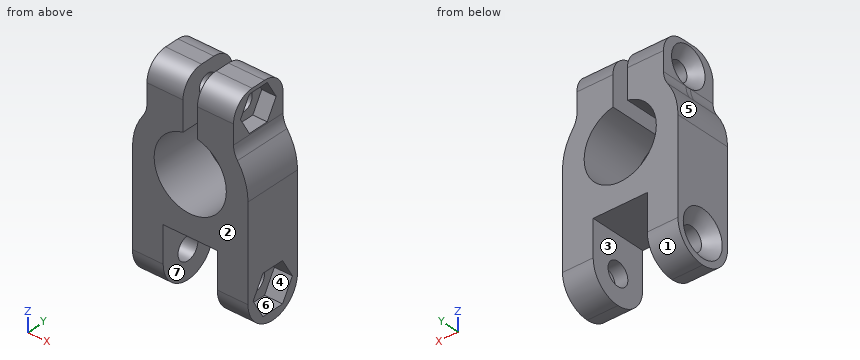
```python
from build123d import *

# Parameters (mm, degrees)
F1_DEPTH = 4
F2_R     = 1.35
F3_DEPTH = 14.001
F4_DEPTH = 2
F5_R     = 1.6
F6_DEPTH = 25
F7_DEPTH = 2.5
F8_SIZE  = 1.35
F9_R     = 3
F10_R    = 3.99999
F11_SIZE = 1.55


# Not quite as in the source:
# - a fillet or chamfer is up to 0.001 mm smaller than in the source, because OpenCascade refuses the exact size
# - a feature names something its author has since deleted; it is built from what else it names


with BuildPart() as f1:
    # F0 (on Front) → F1 (new body, symmetric)
    with BuildSketch(Plane.XZ):
        with BuildLine():
            ThreePointArc((1, 4.8989794856), (0, -5), (-1, 4.8989794856))
            Line((-1, 4.8989794856), (-1, 12))
            Line((-1, 12), (-6, 12))
            Line((-6, 12), (-6, 5.2915026221))
            ThreePointArc((-6, 5.2915026221), (-7.4833147735, 2.8284271247), (-8, 0))
            Line((-8, 0), (-8, -17))
            Line((-8, -17), (-3.75, -17))
            Line((-3.75, -17), (-3.75, -8))
            Line((-3.75, -8), (3.75, -8))
            Line((3.75, -8), (3.75, -17))
            Line((3.75, -17), (8, -17))
            Line((8, -17), (8, 0))
            ThreePointArc((8, 0), (7.4833147735, 2.8284271247), (6, 5.2915026221))
            Line((6, 5.2915026221), (6, 12))
            Line((6, 12), (1, 12))
            Line((1, 12), (1, 4.8989794856))
        make_face()
    extrude(amount=F1_DEPTH, both=True)

    # F2 (on face) → F3 (cut, through all)
    with BuildSketch(Plane.YZ.offset(6)):
        with Locations((0, 9)):
            Circle(F2_R)
    extrude(amount=-F3_DEPTH, mode=Mode.SUBTRACT)

    # F2 (on face) → F4 (cut)
    with BuildSketch(Plane.YZ.offset(6)):
        Polygon((2.8867513459, 9), (1.443375673, 11.5), (-1.443375673, 11.5), (-2.8867513459, 9), (-1.443375673, 6.5), (1.443375673, 6.5), align=None)
        with Locations((0, 9)):
            Circle(F2_R, mode=Mode.SUBTRACT)
    extrude(amount=-F4_DEPTH, mode=Mode.SUBTRACT)

    # F5 (on face) → F6 (cut)
    with BuildSketch(Plane.YZ.offset(8)):
        with Locations((0, -13)):
            Circle(F5_R)
    extrude(amount=-F6_DEPTH, mode=Mode.SUBTRACT)

    # F5 (on face) → F7 (cut)
    with BuildSketch(Plane.YZ.offset(8)):
        Polygon((1.5877132403, -10.25), (-1.5877132403, -10.25), (-3.1754264805, -13), (-1.5877132403, -15.75), (1.5877132403, -15.75), (3.1754264805, -13), align=None)
        with Locations((0, -13)):
            Circle(F5_R, mode=Mode.SUBTRACT)
    extrude(amount=-F7_DEPTH, mode=Mode.SUBTRACT)

    # F8
    f8_edges = [f1.edges().sort_by_distance(p)[0] for p in [
        (-6, -1.35, 9),
    ]]
    chamfer(f8_edges, length=F8_SIZE)

    # F9
    f9_edges = [f1.edges().sort_by_distance(p)[0] for p in [
        (-3.5, -4, 12),
        (3.5, -4, 12),
        (3.5, 4, 12),
        (-3.5, 4, 12),
        (6, 0, 5.291503),
        (-6, 0, 5.291503),
    ]]
    fillet(f9_edges, radius=F9_R)

    # F10 (radius 4 in the source; OpenCascade refuses exactly that, so slightly less here)
    f10_edges = [f1.edges().sort_by_distance(p)[0] for p in [
        (5.875, -4, -17),
        (-5.875, -4, -17),
        (-5.875, 4, -17),
        (5.875, 4, -17),
    ]]
    fillet(f10_edges, radius=F10_R)

    # F11
    f11_edges = [f1.edges().sort_by_distance(p)[0] for p in [
        (-8, -1.6, -13),
    ]]
    chamfer(f11_edges, length=F11_SIZE)


solid = f1.part
```
Here's how the part is built. I have some questions about the finished solid (model axes, mm). Face numbers are marked on the shaded views. A direction names the side the tool comes from. Give positions to 0.01 mm unless a question says otherwise; leave off trailing zeros. Loops run counter-clockwise (first coordinate to the right, second up) from the corner with the lowest first, then second, coordinate; pieces in that order, holes last. Notation, with made-up numbers: M 17,23.5 L 53,23.5 A15 ccw 53,51.5 Z; hole C 55,-14 d2. An arc over 180 degrees is marked long. Use one line per item in the form item = value. Start each with the question number.
Q1. Will these pins go through, and if not, where does the flat tip stop? pin 1 Ø3 at (y, z) = (-0.5, -12.5) entering from +X; pin 2 Ø3 at (y, z) = (-0.5, 9.5) entering from +X; pin 3 Ø2 at (x, y) = (4, -0.5) entering from -Z; pin 4 Ø1.5 at (y, z) = (-2.5, 8.5) entering from +X.
Q2. If we section it at A-A (x = 3): Write out the boundary of the cut face in (y, z), then the cut area to 3 significant figures.
Q3. If we section it at B-B (z = -0.5): Write out the boundary of the cut face in (x, y), then the cut area to 3 significant figures.
Q4. If we section it at D-D (z = -4.5): Write out the boundary of the cut face in (x, y), then the cut area to 3 significant figures.
Q5. I need wall thicknesses on line 1 along X through (y, z) = (-2.5, -10.5); line 2 along Z through (x, y) = (4.2, 0); line 3 along Z through (x, y) = (4.5, -2). Which ranges of each line are inside material? Lowest first, please.
Q6. If we section it at C-C (x = 0): Write out the boundary of the cut face in (y, z).
Q7. Thinking about a two-plate mould opening in Y: for the marked faces 1, 2, 3 and 4, which applies, +Y half, -Y half, draft (parallel to the pull), parting line (faces both ways), or undercut?
Q8. Which directions (+Z, -Z, +X, -X, +Y, -Y) give clear straight access to the entire face, cutting with the end or side of a thin tool? Please do the marked faces 5, 6 and 7.
Taken from the geometry:
q1.pin_1 = 5.5
q1.pin_2 = 4
q1.pin_3 = -17
q1.pin_4 = 6
q2.outline = M -4,-8 L 4,-8 L 4,-4 L -4,-4 Z; M -4,4 L 4,4 L 4,9 A3 ccw 1,12 L -1,12 A3 ccw -4,9 Z; hole C 0,9 d2.7
q2.area = 86.4 mm^2
q3.outline = M -8,-4 L -4.97,-4 L -4.97,4 L -8,4 Z; M 4.97,-4 L 8,-4 L 8,4 L 4.97,4 Z
q3.area = 48.4 mm^2
q4.outline = M -8,-4 L -2.18,-4 L -2.18,4 L -8,4 Z; M 2.18,-4 L 8,-4 L 8,4 L 2.18,4 Z
q4.area = 93.1 mm^2
q5.line_1 = -8 to -3.75, 3.75 to 8
q5.line_2 = -17 to -14.6, -11.4 to -2.71, 2.71 to 6.5, 11.5 to 12
q5.line_3 = -16.46 to -2.18, 2.18 to 7.46, 10.54 to 11.83
q6.outline = M -4,-8 L 4,-8 L 4,-5 L -4,-5 Z
q7.face_1 = +Y half
q7.face_2 = -Y half
q7.face_3 = draft
q7.face_4 = undercut
q8.face_5 = +Z, -X, +Y, -Y
q8.face_6 = +X
q8.face_7 = -Z, +Y, -Y
